Check sheet for the modelled part. Datum: model origin and axes. Units: mm. A direction names the side the tool comes from. Coordinates: 2 decimals unless noted, no trailing zeros. Loops run counter-clockwise (first coordinate to the right, second up) from the corner with the lowest first, then second, coordinate; pieces in that order, holes last. Notation, with made-up numbers: M 9,4 L 50,4 A21 ccw 50,39 Z; hole C 21,69.25 d4. An arc over 180 degrees is marked long. Return JSON: item names as keys, results as strings.
from build123d import *

# Parameters (mm, degrees)
BOSS_EXTRUDE1_DEPTH   = 4
CUT_EXTRUDE1_DEPTH    = 17
BOSS_EXTRUDE2_DEPTH   = 19.5
BOSS_EXTRUDE3_DEPTH   = 4
SKETCH6_W             = 58
SKETCH6_H             = 2
BOSS_EXTRUDE4_DEPTH   = 9
CUT_EXTRUDE2_DEPTH    = 7
FILLET1_R             = 7
BOSS_EXTRUDE5_DEPTH   = 23.5
SKETCH9_W             = 26
SKETCH9_H             = 2
SKETCH9_W_2           = 26.001587477
BOSS_EXTRUDE6_DEPTH   = 9
CUT_EXTRUDE3_DEPTH    = 10
SKETCH11_R            = 1
CUT_EXTRUDE4_DEPTH    = 10
SKETCH12_R            = 2
CUT_EXTRUDE5_DEPTH    = 1.5
SKETCH13_W            = 13.69136931
SKETCH13_H            = 23.795369164
CUT_EXTRUDE6_DEPTH    = 21.5
FILLET2_R             = 2
FILLET2_OF_MIRROR11_R = 2
FILLET3_R             = 6
BOSS_EXTRUDE7_DEPTH   = 7


with BuildPart() as part:
    # Sketch1 → Boss-Extrude1 (new body)
    with BuildSketch(Plane(origin=(0, 0, 0), x_dir=(1, 0, 0), z_dir=(0, 1, 0))):
        with BuildLine():
            ThreePointArc((30.25, 20.5), (33.078427125, 19.328427125), (34.25, 16.5))
            add(Edge.make_bspline(
                [(34.25, 16.5), (37.722666951, -0.526670932), (34.25, -16.5)],
                knots=[0, 0, 0, 0.709821526, 0.709821526, 0.709821526], degree=2))
            ThreePointArc((34.25, -16.5), (33.078427125, -19.328427125), (30.25, -20.5))
            add(Edge.make_bspline(
                [(-30.25, -20.5), (0.344261678, -24.605611324), (30.25, -20.5)],
                knots=[0, 0, 0, 0.814994135, 0.814994135, 0.814994135], degree=2))
            ThreePointArc((-30.25, -20.5), (-33.078427125, -19.328427125), (-34.25, -16.5))
            add(Edge.make_bspline(
                [(-34.25, 16.5), (-37.722666951, -0.526670933), (-34.25, -16.5)],
                knots=[0, 0, 0, 0.709821526, 0.709821526, 0.709821526], degree=2))
            ThreePointArc((-34.25, 16.5), (-33.078427125, 19.328427125), (-30.25, 20.5))
            add(Edge.make_bspline(
                [(-30.25, 20.5), (0.344261678, 24.605611324), (30.25, 20.5)],
                knots=[0, 0, 0, 0.814994135, 0.814994135, 0.814994135], degree=2))
        make_face()
    extrude(amount=BOSS_EXTRUDE1_DEPTH)

    # Sketch2 → Cut-Extrude1 (cut)
    with BuildSketch(Plane(origin=(0, 4, 0), x_dir=(1, 0, 0), z_dir=(0, 1, 0))):
        with BuildLine():
            Line((-3, 0), (-3, -22.530259042))
            add(Edge.make_bspline(
                [(-3, -22.530259042), (0.003385515, -22.572928062), (3, -22.534846829)],
                knots=[0, 0, 0, 1, 1, 1], degree=2))
            Line((3, -22.534846829), (3, 0))
            Line((3, 0), (-3, 0))
        make_face()
    extrude(amount=-CUT_EXTRUDE1_DEPTH, mode=Mode.SUBTRACT)



with BuildPart() as body_2:
    # Sketch3 → Boss-Extrude2 (new body)
    with BuildSketch(Plane(origin=(0, 4, 0), x_dir=(1, 0, 0), z_dir=(0, 1, 0))):
        with BuildLine():
            Line((-29, 20.664354546), (-29, 24.667980394))
            Line((-29, 24.667980394), (29, 24.667980394))
            Line((29, 24.667980394), (29, 20.667980394))
            add(Edge.make_bspline(
                [(29, 20.667980394), (0.316394821, 24.439442983), (-29, 20.664354546)],
                knots=[0, 0, 0, 1, 1, 1], degree=2))
        make_face()
    extrude(amount=BOSS_EXTRUDE2_DEPTH)


with BuildPart() as part_1:
    add(part.part)

    add(body_2.part)  # Boss-Extrude3 merges body 2
    # Sketch4 → Boss-Extrude3 (add)
    with BuildSketch(Plane.XZ.offset(-4)):
        with BuildLine():
            Line((-29.000000006, -20.664354545), (-29, -24.667980394))
            Line((-29, -24.667980394), (29, -24.667980394))
            Line((29, -24.667980394), (29, -20.667980394))
            add(Edge.make_bspline(
                [(29, -20.667980394), (0.316394818, -24.439442983), (-29.000000006, -20.664354545)],
                knots=[0, 0, 0, 1, 1, 1], degree=2))
        make_face()
    extrude(amount=BOSS_EXTRUDE3_DEPTH)

    # Sketch6 → Boss-Extrude4 (add)
    with BuildSketch(Plane(origin=(0, 0, -24.667980394), x_dir=(-1, 0, 0), z_dir=(0, 0, -1))):
        with Locations((0, 22.5)):
            Rectangle(SKETCH6_W, SKETCH6_H)
    extrude(amount=-BOSS_EXTRUDE4_DEPTH)

    # Sketch7 → Cut-Extrude2 (cut)
    with BuildSketch(Plane(origin=(0, 23.5, 0), x_dir=(1, 0, 0), z_dir=(0, 1, 0))):
        with BuildLine():
            Line((-29, 15.667980394), (29, 15.667980394))
            add(Edge.make_bspline(
                [(-29, 15.667980394), (0.2737777, 19.470424078), (29, 15.667980394)],
                knots=[0, 0, 0, 0.915261327, 0.915261327, 0.915261327], degree=2))
        make_face()
    extrude(amount=-CUT_EXTRUDE2_DEPTH, mode=Mode.SUBTRACT)

    # Fillet1
    # the kernel refuses this fillet: 7 mm, written as the material it adds along each edge
    with BuildSketch(Plane(origin=(-29.000000006, 4, -20.664354545), x_dir=(-0.9914665134907249, 0, 0.13036162252191422), z_dir=(0, -1, 0))) as fillet1_piece_1:
        with BuildLine():
            CenterArc((6.441264071, 4.707691972), FILLET1_R, 187.490489673, 34.771943947)
            Line((-0.499001522, 3.795160604), (-0.637806834, 3.776909977))
            Line((-0.637806834, 3.776909977), (-0.138805312, -0.018250627))
            Line((-0.138805312, -0.018250627), (0.000373506, -0.139999502))
            ThreePointArc((0.000373506, -0.139999502), (0.630379223, -0.139159591), (1.157148553, -0.094153839))
            Line((1.157148553, -0.094153839), (1.260758661, 0))
        make_face()
    extrude(amount=4)
    with BuildSketch(Plane(origin=(29, 4, -20.667980394), x_dir=(0.9910909157815452, 0, 0.13318707390470766), z_dir=(0, -1, 0))) as fillet1_piece_2:
        with BuildLine():
            CenterArc((6.428302474, -4.722438864), FILLET1_R, 137.57425577, 34.771944029)
            Line((-0.509333936, -3.790129346), (-0.648086665, -3.771483156))
            Line((-0.648086665, -3.771483156), (-0.138752728, 0.01864619))
            Line((-0.138752728, 0.01864619), (0.000398861, 0.139999432))
            ThreePointArc((0.000398861, 0.139999432), (0.630618203, 0.139101807), (1.157895141, 0.094448777))
            Line((1.157895141, 0.094448777), (1.261236462, 0))
        make_face()
    extrude(amount=4)

    # Sketch8 → Boss-Extrude5 (add)
    with BuildSketch(Plane.XZ):
        with BuildLine():
            add(Edge.make_bspline(
                [(2.999999846, 22.534846831), (16.064348435, 22.368823982), (29, 20.667980394)],
                knots=[0, 0, 0, 0.953900197, 0.953900197, 0.953900197], degree=2))
            Line((29, 20.667980394), (29, 24.667980394))
            Line((29, 24.667980394), (2.999999846, 24.667980394))
            Line((2.999999846, 24.667980394), (2.999999846, 22.534846831))
        make_face()
        with BuildLine():
            Line((-3, 24.667980394), (-29, 24.667980394))
            Line((-29, 24.667980394), (-29, 20.664354545))
            add(Edge.make_bspline(
                [(-29, 20.664354545), (-15.937182308, 22.346460832), (-3, 22.530259042)],
                knots=[0.045651019, 0.045651019, 0.045651019, 1, 1, 1], degree=2))
            Line((-3, 22.530259042), (-3, 24.667980394))
        make_face()
    extrude(amount=-BOSS_EXTRUDE5_DEPTH)

    # Sketch9 → Boss-Extrude6 (add)
    with BuildSketch(Plane.XY.offset(24.667980394)):
        with Locations((-16, 22.5)):
            Rectangle(SKETCH9_W, SKETCH9_H)
        with Locations((16.000793585, 22.5)):
            Rectangle(SKETCH9_W_2, SKETCH9_H)
    extrude(amount=-BOSS_EXTRUDE6_DEPTH)

    # Sketch10 → Cut-Extrude3 (cut)
    with BuildSketch(Plane(origin=(0, 23.5, 0), x_dir=(1, 0, 0), z_dir=(0, 1, 0))):
        with BuildLine():
            Line((-29, -15.667980394), (29.001587323, -15.667980394))
            add(Edge.make_bspline(
                [(-29, -15.667980394), (0.20822973, -18.978019575), (29.001587323, -15.667980394)],
                knots=[0, 0, 0, 0.914206728, 0.914206728, 0.914206728], degree=2))
        make_face()
    extrude(amount=-CUT_EXTRUDE3_DEPTH, mode=Mode.SUBTRACT)

    # Sketch11 → Cut-Extrude4 (cut)
    with BuildSketch(Plane(origin=(0, 4, 0), x_dir=(1, 0, 0), z_dir=(0, 1, 0))):
        with Locations(Location((-9, 14.15, 0), (0, 0, 270))):
            Circle(SKETCH11_R)
        with Locations(Location((-9, -14.15, 0), (0, 0, 270))):
            Circle(SKETCH11_R)
    cut_extrude4 = extrude(amount=-CUT_EXTRUDE4_DEPTH, mode=Mode.SUBTRACT)

    # Sketch12 → Cut-Extrude5 (cut)
    with BuildSketch(Plane(origin=(0, 4, 0), x_dir=(1, 0, 0), z_dir=(0, 1, 0))):
        with Locations(Location((-9, 14.15, 0), (0, 0, 270))):
            Circle(SKETCH12_R)
        with Locations(Location((-9, -14.15, 0), (0, 0, 270))):
            Circle(SKETCH12_R)
    cut_extrude5 = extrude(amount=-CUT_EXTRUDE5_DEPTH, mode=Mode.SUBTRACT)

    # Mirror10: Cut-Extrude4, Cut-Extrude5 across plane
    add(cut_extrude4.mirror(Plane.ZY), mode=Mode.SUBTRACT)
    add(cut_extrude5.mirror(Plane.ZY), mode=Mode.SUBTRACT)

    # Sketch13 → Cut-Extrude6 (cut)
    with BuildSketch(Plane(origin=(0, 4, 0), x_dir=(1, 0, 0), z_dir=(0, 1, 0))):
        with Locations((-20.556344598, -0.164609633)):
            Rectangle(SKETCH13_W, SKETCH13_H)
    cut_extrude6 = extrude(amount=-CUT_EXTRUDE6_DEPTH, mode=Mode.SUBTRACT)

    # Fillet2
    fillet2_edges = [part_1.edges().sort_by_distance(p)[0] for p in [
        (-13.710659943, 2, -11.733074949),
        (-13.710659943, 2, 12.062294215),
        (-27.402029253, 2, 12.062294215),
        (-27.402029253, 2, -11.733074949),
    ]]
    fillet(fillet2_edges, radius=FILLET2_R)

    # Mirror11: Cut-Extrude6 across plane
    add(cut_extrude6.mirror(Plane.ZY), mode=Mode.SUBTRACT)

    # Fillet2 of Mirror11
    fillet2_of_mirror11_edges = [part_1.edges().sort_by_distance(p)[0] for p in [
        (13.710659959, 2, -11.73307493),
        (13.710659926, 2, 12.062294234),
        (27.402029236, 2, 12.062294253),
        (27.40202927, 2, -11.733074911),
    ]]
    fillet(fillet2_of_mirror11_edges, radius=FILLET2_OF_MIRROR11_R)

    # Fillet3
    # the kernel refuses this fillet: 6 mm, written as the material it adds along each edge
    with BuildSketch(Plane(origin=(-29, 0, 20.664354545), x_dir=(-0.9914665134873252, 0, -0.13036162254777076), z_dir=(0, 1, 0))) as fillet3_piece_1:
        with BuildLine():
            CenterArc((5.492355455, 4.253655913), FILLET3_R, 187.490489592, 37.658462004)
            Line((-0.456443626, 3.471486178), (-0.575419608, 3.455842783))
            Line((-0.575419608, 3.455842783), (-0.118975982, -0.015643395))
            Line((-0.118975982, -0.015643395), (0.000320148, -0.119999573))
            ThreePointArc((0.000320148, -0.119999573), (0.630379241, -0.119159591), (1.176126731, -0.085073118))
            Line((1.176126731, -0.085073118), (1.260758667, 0))
        make_face()
    extrude(amount=4)
    with BuildSketch(Plane(origin=(29, 0, 20.667980394), x_dir=(0.9910909157697056, 0, -0.1331870739928102), z_dir=(0, 1, 0))) as fillet3_piece_2:
        with BuildLine():
            CenterArc((5.480691848, -4.265699972), FILLET3_R, 134.68773779, 37.658462005)
            Line((-0.465853647, -3.466577528), (-0.584784557, -3.450595079))
            Line((-0.584784557, -3.450595079), (-0.11893091, 0.015982449))
            Line((-0.11893091, 0.015982449), (0.000341881, 0.119999513))
            ThreePointArc((0.000341881, 0.119999513), (0.630618207, 0.119101807), (1.176847354, 0.085313999))
            Line((1.176847354, 0.085313999), (1.261236462, 0))
        make_face()
    extrude(amount=4)

    # Sketch14 → Boss-Extrude7 (add)
    with BuildSketch(Plane.XZ):
        with BuildLine():
            Line((-31.25, 16.5), (-34.25, 16.5))
            add(Edge.make_bspline(
                [(-34.25, -16.5), (-37.722666951, 0.526670933), (-34.25, 16.5)],
                knots=[0, 0, 0, 1, 1, 1], degree=2))
            Line((-34.25, -16.5), (-31.25, -16.5))
            add(Edge.make_bspline(
                [(-31.25, -16.5), (-34.771209982, 0.410301421), (-31.25, 16.5)],
                knots=[0, 0, 0, 1, 1, 1], degree=2))
        make_face()
    boss_extrude7 = extrude(amount=-BOSS_EXTRUDE7_DEPTH)

    # Mirror12: Boss-Extrude7 across plane
    add(boss_extrude7.mirror(Plane.ZY))


solid = part_1.part
1) Go/stop test with flat-tipped pins: pin 1 Ø2.5 at (x, z) = (-34.5, 5) entering from +Y; pin 2 Ø4.5 at (y, z) = (2, 4.5) entering from -X; pin 3 Ø10 at (x, z) = (-10, 6.5) entering from +Y. Record where each tip stops, or that it passes through.
Answers:
{"pin 1": "y = 7", "pin 2": "x = -35.96", "pin 3": "y = 4"}
2) Draft check along Z on faces 1 (the face through (-29.31, 2.03, -22.43)), 2 (the face through (-26.8, 1.97, 11.49)), 3 (the face through (33.109, 1.972, 19.297)). Enter one of: +Z half, -Z half, draft (parallel to the pull), parting line (faces both ways), or undercut.
Answers:
{"face 1": "-Z half", "face 2": "undercut", "face 3": "+Z half"}
3) Section check B-B on x = -9. Count the separate pieces of the cut face and the enclosed holes in it, then the cut area to 3 significant figures.
Answers:
{"separate pieces": "3", "enclosed holes": "0", "area": "286 mm²"}
4) Scan lines: line 1 along Z through (x, y) = (9, 3.7); line 2 along Z through (x, y) = (17.5, 2); line 3 along X through (y, z) = (22, 22). Record each from-to range of solid material in increasing order. Write a range as [from, to].
Answers:
{"line 1": "[-24.67, -16.15], [-12.15, 12.15], [16.15, 24.67]", "line 2": "[-24.67, -11.73], [12.06, 24.67]", "line 3": "[-29, -3], [3, 29]"}
5) Set-up check for faces 4 (the face through (-7.017, 3.26, -14.41)), 5 (the face through (-16, 21.5, 19)), 6 (the face through (0.4, 0, -0.5)), 7 (the face through (0, 12, -24.668)), 8 (the face through (-13.711, 2, 0)): record each of +Z, -Z, +X, -X, +Y, -Y from which the full face is reachable in a straight line by a thin tool's end or side.
Answers:
{"face 4": "+Y", "face 5": "none", "face 6": "+Z, -Z, +X, -X, -Y", "face 7": "-Z, +X, -X, +Y, -Y", "face 8": "+Y, -Y"}
6) Section check A-A on z = 19. Record the cut outline in (x, y).
Answers:
{"outline": "M -33.37,0 L -3,0 L -3,4 L -33.37,4 Z; M -29,21.5 L -3,21.5 L -3,23.5 L -29,23.5 Z; M 3,0 L 33.37,0 L 33.37,4 L 3,4 Z; M 3,21.5 L 29,21.5 L 29,23.5 L 3,23.5 Z"}
